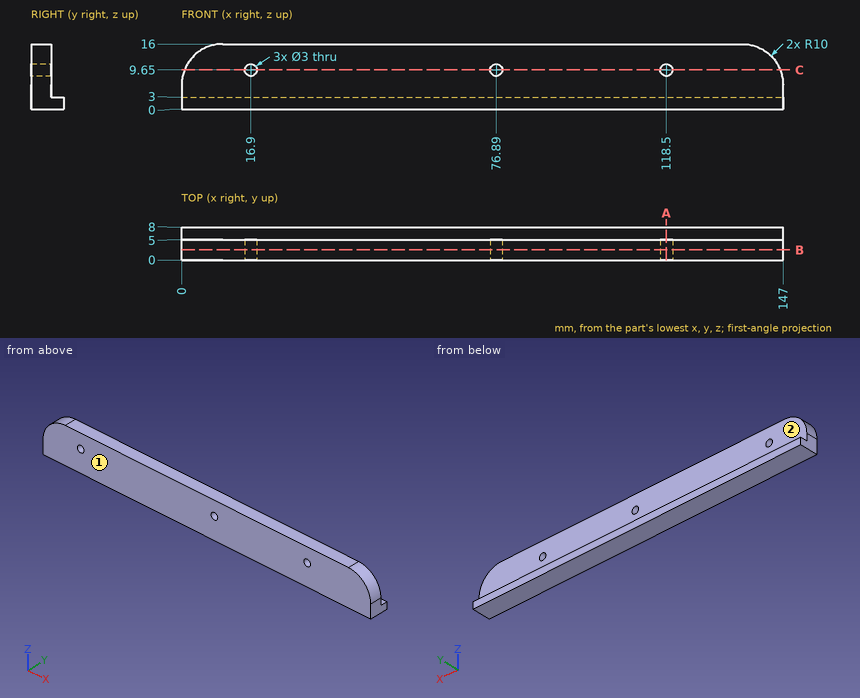
Design review of the part shown in the three views and the two pictorial views. Dimensions are in mm from the part's minimum x, y and z. A direction names the side the tool comes from. Give positions to 0.01 mm unless a question says otherwise; leave off trailing zeros. Loops run counter-clockwise (first coordinate to the right, second up) from the corner with the lowest first, then second, coordinate; pieces in that order, holes last. Notation, with made-up numbers: (-19, 40) -> (27, 40) arc R20 ccw to (27, 53) -> close; hole circle Ø10 at (52.25, 63.25). An arc over 180 degrees is marked (long way). Put each result on its own line as item: value. Start each with the question number.
1. Clearance check with flat-ended pins moving along their axes: P1, Ø1, axis at y = 5, z = 9.5, coming from the +X side; P2, Ø6, axis at x = 62.5, z = 6.5, coming from the +Y side; P3, Ø3, axis at y = 4.5, z = 13, coming from the -X side; P4, Ø2.5, axis at x = 16.9, z = 9.65, coming from the -Y side. State where each tip first meets the part, or that it passes through.
2. Wall thickness on probe 1 along Z at (x, y) = (16.9, 1.65); probe 2 along X at (y, z) = (1.5, 9.65); probe 3 along X at (y, z) = (2.75, 9.25): over which ranges is each line inside the solid? List them lowest first.
3. We need section C-C on z = 9.65. State the section outline as (x, y) points, then the cut area to 3 significant figures.
4. For the marked faces 1 and 2, list the 3-axis set-ups (+Z, -Z, +X, -X, +Y, -Y) from which the entire face can be reached by the end or side of a thin tool; tool diameter is ignored.
5. We need section B-B on y = 2.5. State the section outline as (x, z) points, then the cut area to 3 significant figures.
6. We need section A-A on x = 118.5. State the section outline as (y, z) points, then the cut area to 3 significant figures.
Determined:
1. P1: x = 146.54
1. P2: y = 5
1. P3: x = 1.65
1. P4: through
2. probe 1: 0 to 8.15, 11.15 to 16
2. probe 2: 0.69 to 15.4, 18.4 to 75.39, 78.39 to 117, 120 to 146.31
2. probe 3: 0.54 to 15.45, 18.35 to 75.44, 78.34 to 117.05, 119.95 to 146.46
3. outline: (0.69, 0) -> (15.4, 0) -> (15.4, 5) -> (0.69, 5) -> close; (18.4, 0) -> (75.39, 0) -> (75.39, 5) -> (18.4, 5) -> close; (78.39, 0) -> (117, 0) -> (117, 5) -> (78.39, 5) -> close; (120, 0) -> (146.31, 0) -> (146.31, 5) -> (120, 5) -> close
3. area: 683 mm^2
4. face 1: +Z, -Z, +X, -X, -Y
4. face 2: +Z, +X, -X, +Y
5. outline: (0, 0) -> (147, 0) -> (147, 6) arc R10 ccw to (137, 16) -> (10, 16) arc R10 ccw to (0, 6) -> close; hole circle Ø3 at (16.9, 9.65); hole circle Ø3 at (76.89, 9.65); hole circle Ø3 at (118.5, 9.65)
5. area: 2,290 mm^2
6. outline: (0, 0) -> (8, 0) -> (8, 3) -> (5, 3) -> (5, 8.15) -> (0, 8.15) -> close; (0, 11.15) -> (5, 11.15) -> (5, 16) -> (0, 16) -> close
6. area: 74.0 mm^2
